```python
from build123d import *

# Parameters (mm, degrees)
BOSS_EXTRUDE1_DEPTH = 180
SKETCH2_W           = 120
SKETCH2_H           = 120
BOSS_EXTRUDE2_DEPTH = 10
SKETCH3_R           = 5
CUT_EXTRUDE1_DEPTH  = 10
SKETCH4_W           = 110
SKETCH4_H           = 30
CUT_EXTRUDE2_DEPTH  = 10
SKETCH5_W           = 30
SKETCH5_H           = 5
BOSS_EXTRUDE3_DEPTH = 30


with BuildPart() as part:
    # Sketch1 → Boss-Extrude1 (new body)
    with BuildSketch(Plane.XY):
        Polygon((-60, 60), (60, 60), (60, -60), (40, -60), (40, -55), (55, -55), (55, 55), (-55, 55), (-55, -55), (-40, -55), (-40, -60), (-60, -60), align=None)
    extrude(amount=BOSS_EXTRUDE1_DEPTH)

    # Sketch2 → Boss-Extrude2 (add)
    with BuildSketch(Plane.XY.offset(180)):
        Rectangle(SKETCH2_W, SKETCH2_H)
    extrude(amount=BOSS_EXTRUDE2_DEPTH)

    # Sketch3 → Cut-Extrude1 (cut)
    with BuildSketch(Plane.XY.offset(190)):
        Circle(SKETCH3_R)
    extrude(amount=-CUT_EXTRUDE1_DEPTH, mode=Mode.SUBTRACT)

    # Sketch4 → Cut-Extrude2 (cut)
    with BuildSketch(Plane(origin=(0, 60, 0), x_dir=(1, 0, 0), z_dir=(0, 1, 0))):
        with Locations((0, -165)):
            Rectangle(SKETCH4_W, SKETCH4_H)
    extrude(amount=-CUT_EXTRUDE2_DEPTH, mode=Mode.SUBTRACT)

    # Sketch5 → Boss-Extrude3 (add)
    with BuildSketch(Plane(origin=(0, 60, 0), x_dir=(1, 0, 0), z_dir=(0, 1, 0))):
        with Locations((45, -69.201770824)):
            Rectangle(SKETCH5_W, SKETCH5_H)
    extrude(amount=BOSS_EXTRUDE3_DEPTH)


solid = part.part
```
Read the model definition and answer for the solid it produces. Units are mm, in the model's axes. A direction names the side the tool comes from. Give positions to 0.01 mm unless a question says otherwise; leave off trailing zeros. Order: outer loops, then holes, each group sorted by start corner. A loop starts at its lowest first (then second) coordinate and runs counter-clockwise, first axis right, second up.
(1) For faces 5 (the flat face through (45, 75, 66.702)), 6 (the flat face through (40, -58, 89)), 7 (the flat face through (30, 75, 69)), 8 (the flat face through (45, 75, 71.702)), 9 (the flat face through (47, -55, 89)), determine the directions among +Z, -Z, +X, -X, +Y, -Y from which every point of the face is accessible in a straight line to the end or side of a thin tool.
(2) Given pin 1 (24 mm diameter, centred on x = 50.5, y = 75.5, fed in from +Z); pin 2 (2 mm diameter, centred on x = 38, y = 6, fed in from -Z); pin 3 (12 mm diameter, centred on x = 49, z = 134.5, fed in from +Y), each flat-ended and moving along its own axis, determine where each tip first touches the part or whether it passes through.
(3) Find section D-D (x = -48.5). Give the vertices of the cut face in (y, z).
(4) Straight lines are drawn through the part: L1, parallel to X at y = -1.5, z = 52.5; L2, parallel to Y at x = 0, z = 183. For each, find the intervals that lie inside material, in ascending order.
(5) Find section A-A (y = 0). Give the vertices of the cut face in (x, z).
(6) For a pull along Y with two mould halves and no side action, classify faces 1 (the cylindrical face through (-1.08, -4.88, 185.07)), 2 (the flat face through (-40.3, -60, 108.6)), 3 (the flat face through (-55, 3, 91)), 4 (the flat face through (-60, -1, 94)) as released by +Y, released by -Y, zero draft, split by the parting line, or undercut.
(7) Find section C-C (z = 169). Give the vertices of the cut face in (x, y), plus the area to 3 significant figures.
(8) Find section B-B (x = 0). Give the vertices of the cut face in (y, z).
Result sheet:
1. face 5: -Z, +X, -X, +Y
1. face 6: -Z, -Y
1. face 7: +Z, -Z, -X, +Y
1. face 8: +Z, +X, -X, +Y
1. face 9: -Z
2. pin 1: stops at z = 71.7
2. pin 2: stops at z = 180
2. pin 3: stops at y = 60
3. outline: (-60, 0) - (-55, 0) - (-55, 180) - (60, 180) - (60, 190) - (-60, 190) - close; (55, 0) - (60, 0) - (60, 150) - (55, 150) - close
4. L1: x = -60 to -55, 55 to 60
4. L2: y = -60 to -5, 5 to 60
5. outline: (-60, 0) - (-55, 0) - (-55, 180) - (-5, 180) - (-5, 190) - (-60, 190) - close; (5, 180) - (55, 180) - (55, 0) - (60, 0) - (60, 190) - (5, 190) - close
6. face 1: undercut
6. face 2: released by -Y
6. face 3: undercut
6. face 4: zero draft
7. outline: (-60, -60) - (-40, -60) - (-40, -55) - (-55, -55) - (-55, 60) - (-60, 60) - close; (40, -60) - (60, -60) - (60, 60) - (55, 60) - (55, -55) - (40, -55) - close
7. area: 1,350 mm2
8. outline: (-60, 180) - (-5, 180) - (-5, 190) - (-60, 190) - close; (5, 180) - (60, 180) - (60, 190) - (5, 190) - close; (55, 0) - (60, 0) - (60, 150) - (55, 150) - close
